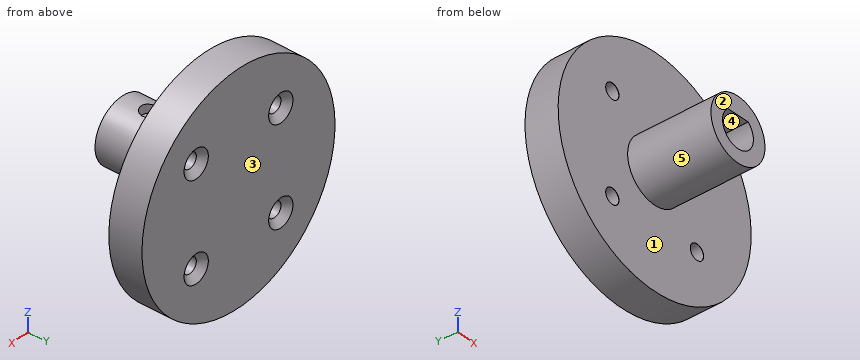
from build123d import *

# Parameters (mm, degrees)
SKETCH1_R                                      = 25
BOSS_EXTRUDE1_DEPTH                            = 7.5
CSK_FOR_M3_FLAT_HEAD_MACHINE_SCREW1_AT_2_COUNT = 2
CSK_FOR_M3_FLAT_HEAD_MACHINE_SCREW1_AT_2_PITCH = 21.920310217
CSK_FOR_M3_FLAT_HEAD_MACHINE_SCREW1_AT_3_COUNT = 2
CSK_FOR_M3_FLAT_HEAD_MACHINE_SCREW1_AT_3_PITCH = 31
CSK_FOR_M3_FLAT_HEAD_MACHINE_SCREW1_AT_4_COUNT = 2
CSK_FOR_M3_FLAT_HEAD_MACHINE_SCREW1_AT_4_PITCH = 21.920310217
SKETCH6_R                                      = 7
BOSS_EXTRUDE2_DEPTH                            = 18.85
SKETCH7_R                                      = 1
CUT_EXTRUDE1_DEPTH                             = 10.5
SKETCH11_R                                     = 1.9
CUT_EXTRUDE2_DEPTH                             = 2


with BuildPart() as part:
    # Sketch1 → Boss-Extrude1 (new body)
    with BuildSketch(Plane(origin=(0, 0, 0), x_dir=(1, 0, 0), z_dir=(0, 1, 0))):
        with Locations(Location((0, 0, 0), (0, 0, 270))):
            Circle(SKETCH1_R)
    extrude(amount=BOSS_EXTRUDE1_DEPTH)

    # Sketch5 → CSK for M3 Flat Head Machine Screw1 (revolve, cut)
    with BuildSketch(Plane(origin=(-10.960155108, 7.5, -10.960155108), x_dir=(0, 0, 1), z_dir=(1, 0, 0))):
        Polygon((0, 0), (0, 7.5), (1.725, 7.5), (1.7, 7.475), (1.7, 1.45), (3.15, 0), align=None)
    csk_for_m3_flat_head_machine_screw1 = revolve(axis=Axis((-10.960155108, 13.85, -10.960155108), (0, -1, 0)), mode=Mode.SUBTRACT)

    # CSK for M3 Flat Head Machine Screw1 at 2: CSK for M3 Flat Head Machine Screw1 ×2
    with Locations(*[(i * CSK_FOR_M3_FLAT_HEAD_MACHINE_SCREW1_AT_2_PITCH, 0, 0) for i in range(1, CSK_FOR_M3_FLAT_HEAD_MACHINE_SCREW1_AT_2_COUNT)]):
        add(csk_for_m3_flat_head_machine_screw1, mode=Mode.SUBTRACT)

    # CSK for M3 Flat Head Machine Screw1 at 3: CSK for M3 Flat Head Machine Screw1 ×2
    with Locations(*[Vector(0.7071067811865475, 0, 0.7071067811865476) * (i * CSK_FOR_M3_FLAT_HEAD_MACHINE_SCREW1_AT_3_PITCH) for i in range(1, CSK_FOR_M3_FLAT_HEAD_MACHINE_SCREW1_AT_3_COUNT)]):
        add(csk_for_m3_flat_head_machine_screw1, mode=Mode.SUBTRACT)

    # CSK for M3 Flat Head Machine Screw1 at 4: CSK for M3 Flat Head Machine Screw1 ×2
    with Locations(*[(0, 0, i * CSK_FOR_M3_FLAT_HEAD_MACHINE_SCREW1_AT_4_PITCH) for i in range(1, CSK_FOR_M3_FLAT_HEAD_MACHINE_SCREW1_AT_4_COUNT)]):
        add(csk_for_m3_flat_head_machine_screw1, mode=Mode.SUBTRACT)

    # Sketch6 → Boss-Extrude2 (add)
    with BuildSketch(Plane.XZ):
        with Locations(Location((0, 0, 0), (0, 0, 90))):
            Circle(SKETCH6_R)
        with BuildLine():
            Line((-2.645751311, 3), (2.645751311, 3))
            ThreePointArc((2.645751311, 3), (0, -4), (-2.645751311, 3))
        make_face(mode=Mode.SUBTRACT)
    extrude(amount=BOSS_EXTRUDE2_DEPTH)

    # Sketch7 → Cut-Extrude1 (cut)
    with BuildSketch(Plane.XY):
        with Locations(Location((0, -12.6, 0), (0, 0, 180))):
            Circle(SKETCH7_R)
    extrude(amount=CUT_EXTRUDE1_DEPTH, mode=Mode.SUBTRACT)

    # Sketch11 → Cut-Extrude2 (cut)
    with BuildSketch(Plane.XY.offset(7)):
        with Locations((0, -12.6)):
            Circle(SKETCH11_R)
    extrude(amount=-CUT_EXTRUDE2_DEPTH, mode=Mode.SUBTRACT)


solid = part.part
Here's how the part is built. I have some questions about the finished solid (model axes, mm). Face numbers are marked on the shaded views. A direction names the side the tool comes from. Give positions to 0.01 mm unless a question says otherwise; leave off trailing zeros. Order: outer loops, then holes, each group sorted by start corner. A loop starts at its lowest first (then second) coordinate and runs counter-clockwise, first axis right, second up. Notation, with made-up numbers: (44.25, -36) -> (95.25, -36) arc R18 cw to (95.25, -8) -> close; hole circle Ø2 at (81.25, 4.5). An arc over 180 degrees is marked (long way). One line per item, written item: value. Start each with the question number.
1. For the marked faces 1 and 2, which set-ups out of +Z, -Z, +X, -X, +Y, -Y let a thin tool reach every point of the face, with its end or its side?
2. Imagine slicing it at D-D, the plane y = 4. List the corners of the cut face in (x, z) for me.
3. We'd pull the mould along Z, two halves only. Please class the marked faces 3, 4 and 5: released by +Z, released by -Z, zero draft, split by the parting line, or undercut.
4. Imagine slicing it at C-C, the plane y = -12.6. List the corners of the cut face in (x, z) for me, plus the area to 3 significant figures.
5. Will these pins go through, and if not, where does the flat tip stop? pin 1 Ø4 at (y, z) = (-13.5, -5) entering from +X; pin 2 Ø3 at (x, z) = (7, 6) entering from -Y; pin 3 Ø1.1 at (x, y) = (-0.5, -13.5) entering from +Z; pin 4 Ø2.5 at (x, z) = (-10.96, -10.96) entering from +Y.
6. Imagine slicing it at A-A, the plane x = 0. List the corners of the cut face in (y, z) for me, plus the area to 3 significant figures.
7. Imagine slicing it at B-B, the plane z = 0. List the corners of the cut face in (x, y) for me, plus the area to 3 significant figures.
8. I need wall thicknesses on probe 1 along Y at (x, z) = (0, 5.8); probe 2 along Y at (x, z) = (0, 4); probe 3 along Y at (x, z) = (21, -1.5). Which ranges of each line are inside material? Lowest first, please. Write a range as from..to.
Values follow:
1. face 1: -Y
1. face 2: +Z, -Z, +X, -X, -Y
2. outline: circle Ø50 at (0, 0); hole circle Ø3.4 at (-10.96, -10.96); hole circle Ø3.4 at (-10.96, 10.96); hole circle Ø3.4 at (10.96, -10.96); hole circle Ø3.4 at (10.96, 10.96)
3. face 3: zero draft
3. face 4: undercut
3. face 5: split by the parting line
4. outline: (-2.65, 3) -> (-1, 3) -> (-1, 5) -> (-1.9, 5) -> (-1.9, 6.74) arc R7 ccw (long way) to (1.9, 6.74) -> (1.9, 5) -> (1, 5) -> (1, 3) -> (2.65, 3) arc R4 cw (long way) to start
4. area: 96.0 mm2
5. pin 1: stops at x = 6.32
5. pin 2: stops at y = 0
5. pin 3: stops at z = 5
5. pin 4: passes through
6. outline: (-18.85, -7) -> (0, -7) -> (0, -25) -> (7.5, -25) -> (7.5, 25) -> (0, 25) -> (0, 7) -> (-10.7, 7) -> (-10.7, 5) -> (-11.6, 5) -> (-11.6, 3) -> (0, 3) -> (0, -4) -> (-18.85, -4) -> close; (-18.85, 3) -> (-13.6, 3) -> (-13.6, 5) -> (-14.5, 5) -> (-14.5, 7) -> (-18.85, 7) -> close
6. area: 495 mm2
7. outline: (-25, 0) -> (-7, 0) -> (-7, -18.85) -> (-4, -18.85) -> (-4, 0) -> (4, 0) -> (4, -18.85) -> (7, -18.85) -> (7, 0) -> (25, 0) -> (25, 7.5) -> (-25, 7.5) -> close
7. area: 488 mm2
8. probe 1: y = -18.85..-14.5, -10.7..7.5
8. probe 2: y = -18.85..-13.6, -11.6..7.5
8. probe 3: y = 0..7.5
